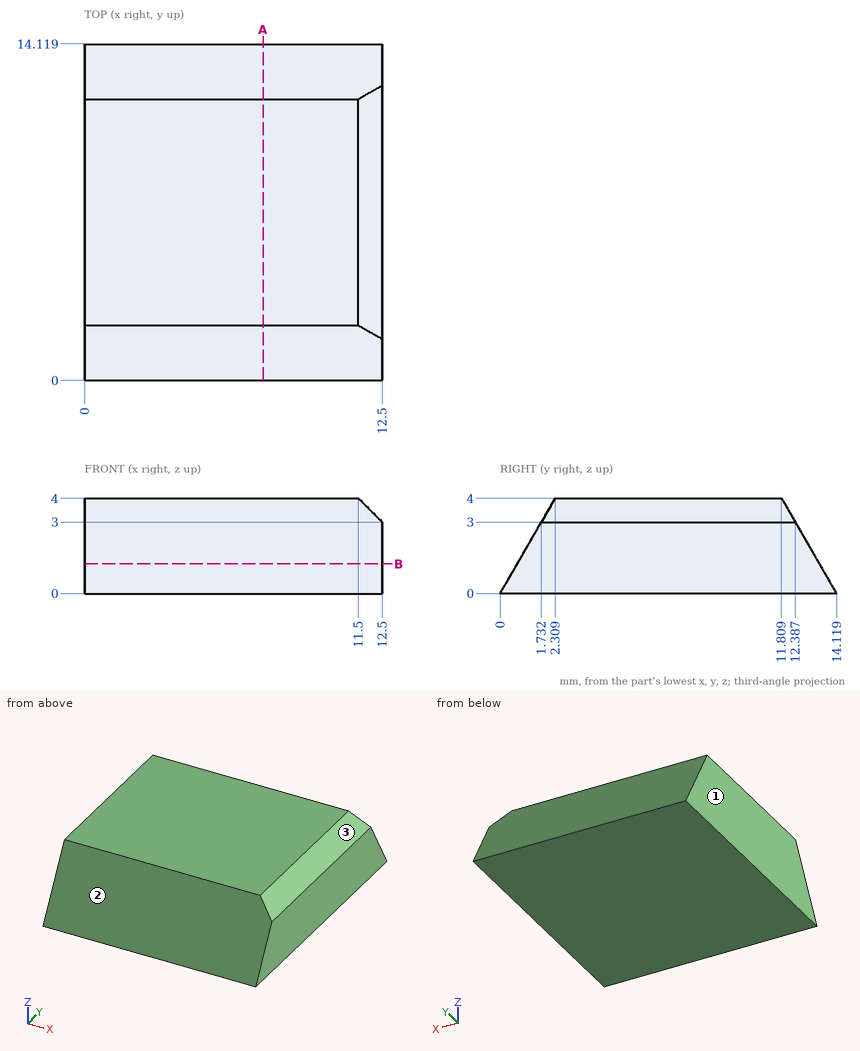
Check sheet for the drawn part. Datum: minimum x, y, z corner. Units: mm. Coordinates: 2 decimals unless noted, no trailing zeros. Order: outer loops, then holes, each group sorted by start corner. A loop starts at its lowest first (then second) coordinate and runs counter-clockwise, first axis right, second up. Notation, with made-up numbers: (25.5, 2.5) - (64.5, 2.5) arc R27 ccw to (64.5, 29.5) - close; hole circle Ø7 at (1.5, 57.25). An arc over 180 degrees is marked (long way). Return JSON: item names as keys, results as strings.
(1) Thickness scan on line 1 along Y through (x, z) = (4, 3.75) (1 decimal); line 2 along Y through (x, z) = (9, 3.2); line 3 along X through (y, z) = (4.5, 3.7). Record the ranges inside material, lowest first.
Filled sheet:
{"line 1": "y = 2.2 to 12", "line 2": "y = 1.85 to 12.27", "line 3": "x = 0 to 11.8"}
(2) Section check A-A, the plane x = 7.5. Record the cut outline in (y, z).
Filled sheet:
{"outline": "(0, 0) - (14.12, 0) - (11.81, 4) - (2.31, 4) - close"}
(3) Go/stop test with flat-tipped pins: pin 1 (1.5 mm diameter, centred on x = 8, z = 3.5, fed in from -Y); pin 2 (1 mm diameter, centred on x = 2, z = 2.5, fed in from -Y) (1 decimal); pin 3 (1.5 mm diameter, centred on x = 3.5, z = 1, fed in from +Y) (1 decimal). Record where each tip stops, or that it passes through.
Filled sheet:
{"pin 1": "stops at y = 1.59", "pin 2": "stops at y = 1.2", "pin 3": "stops at y = 14"}
(4) Mould release check, pull along X, two halves, no side actions. Record for the marked faces 1, 2 and 3: pulls with the +X half, pulls with the -X half, needs draft (parallel to the pull), parting line crosses it, or undercut.
Filled sheet:
{"face 1": "pulls with the -X half", "face 2": "needs draft", "face 3": "pulls with the +X half"}
(5) Section check B-B, the plane z = 1.25. Record the cut outline in (x, y).
Filled sheet:
{"outline": "(0, 0.72) - (12.5, 0.72) - (12.5, 13.4) - (0, 13.4) - close"}
